Autodesk Inventor part; units mm, degrees
ref_plane "YZ Plane" through (0, 0, 0) normal (1, 0, 0) x (0, 1, 0)
ref_plane "XZ Plane" through (0, 0, 0) normal (0, 1, 0) x (-1, 0, 0)
ref_plane "XY Plane" through (0, 0, 0) normal (0, 0, 1) x (1, 0, 0)
sketch "スケッチ1" plane through (0, 0, 0) normal (1, 0, 0) x (0, 1, 0)
  circle A0 centre (0, 0) radius 2.5
  dimension "d0" = 5
extrude "押し出し1" add sketch "スケッチ1" along normal blind 1.25
sketch "スケッチ3" plane through (1.25, 0, 0) normal (1, 0, 0) x (0, 0, -1)
  circle A0 centre (0, 0) radius 1
  dimension "d6" = 2
extrude "押し出し3" add sketch "スケッチ3" along normal blind 2
mirror "ミラー1" about plane through (0, 0, 0) normal (-1, 0, 0) of "押し出し1", "押し出し3"
properties part number "roller"
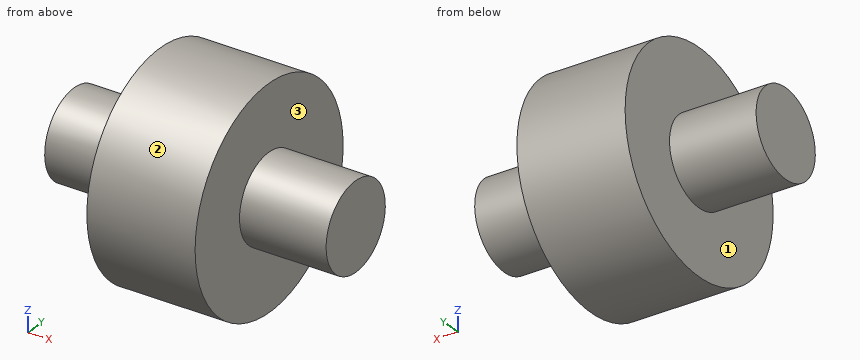
Source: CAD feature listing. Evaluate the final solid. Frame: model axes, mm. Face numbers are marked on the shaded views. A direction names the side the tool comes from. Coordinates: 2 decimals unless noted, no trailing zeros. Order: outer loops, then holes, each group sorted by start corner. A loop starts at its lowest first (then second) coordinate and runs counter-clockwise, first axis right, second up. Notation, with made-up numbers: M 74.5,-27.5 L 116.5,-27.5 A12 ccw 116.5,-4.5 Z; hole C 25,-15 d4. An arc over 180 degrees is marked long. Write each question's results on one line, items separated by ' | '. Start each with the question number.
1. Section D-D, the plane x = -1. Return the cut outline in (y, z).
2. Section A-A, the plane y = 0. Return the cut outline in (x, z).
3. Section C-C, the plane x = -2.5. Return the cut outline in (y, z), then the cut area to 3 significant figures.
4. Material intervals for L1, parallel to X at y = -0.1, z = -1.45; L2, parallel to Z at x = 0.75, y = -0.3; L3, parallel to Y at x = 0.5, z = 1.35, sorted ascending.
5. Reachability of the marked faces 1, 2 and 3 from +Z, -Z, +X, -X, +Y, -Y: full face, straight path, thin tool, end or side. Return the list, or none.
6. Pin query (flat end, axial travel): pin 1 (1.5 mm diameter, centred on x = -2.5, z = -1, fed in from -Y). Return the tip coordinate at first contact, or that it passes through.
Solution:
1) outline: C 0,0 d5
2) outline: M -3.25,-1 L -1.25,-1 L -1.25,-2.5 L 1.25,-2.5 L 1.25,-1 L 3.25,-1 L 3.25,1 L 1.25,1 L 1.25,2.5 L -1.25,2.5 L -1.25,1 L -3.25,1 Z
3) outline: C 0,0 d2 | area: 3.14 mm²
4) L1: -1.25 to 1.25 | L2: -2.48 to 2.48 | L3: -2.1 to 2.1
5) face 1: -X | face 2: +X, -X | face 3: +X
6) pin 1: y = -0.97
